Design review of the part shown in the three views and the two pictorial views. Dimensions are in mm from the part's minimum x, y and z. Round coordinates to 2 decimals unless told otherwise and drop trailing zeros. Loops run counter-clockwise (first coordinate to the right, second up) from the corner with the lowest first, then second, coordinate; pieces in that order, holes last. Notation, with made-up numbers: M -4.5,-39 L 42.5,-39 A28 cw 42.5,-17 Z; hole C 84,51.5 d7. An arc over 180 degrees is marked long. One line per question, with ' | ' between items. Start each with the question number.
1) We need section A-A (x = 17.9). Give the boundary of the cut face in (y, z), and give its area (3 significant figures).
2) For pin 1 Ø2 at (x, y) = (13.5, 39.5) entering from -Z; pin 2 Ø2 at (x, y) = (17, 43) entering from -Z; pin 3 Ø5 at (x, z) = (25, 10.5) entering from -Y; pin 4 Ø8 at (x, y) = (31.5, 19.5) entering from +Z, all flat-tipped, find the tip position at first contact; note any pin that passes through.
3) We need section D-D (x = 2). Give the boundary of the cut face in (y, z), and give its area (3 significant figures).
4) For probe 1 along Z at (x, y) = (17.9, 25.5); probe 2 along X at (y, z) = (44, 19); probe 3 along X at (y, z) = (21, 17), list the stretches that pass through material, from the lowest coordinate up. Write a range as from..to.
5) Mouldability with a two-part tool opening along Z and no side actions: class the marked faces 1, 2 and 3 as pulls with the +Z half, pulls with the -Z half, needs draft (parallel to the pull), parting line crosses it, or undercut.
6) We need section C-C (y = 31). Give the boundary of the cut face in (x, z), and give its area (3 significant figures).
7) We need section B-B (z = 17.9). Give the boundary of the cut face in (x, y).
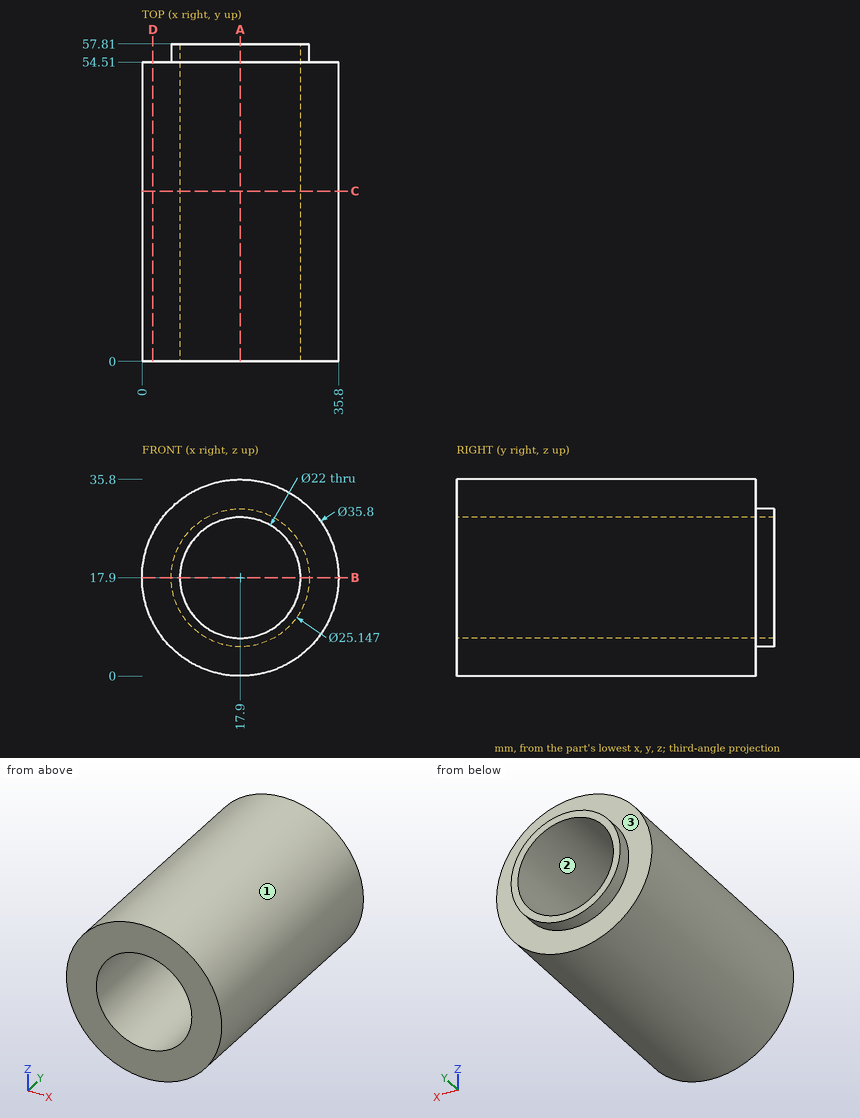
Answers below:
1) outline: M 0,0 L 54.51,0 L 54.51,5.33 L 57.81,5.33 L 57.81,6.9 L 0,6.9 Z; M 0,28.9 L 57.81,28.9 L 57.81,30.47 L 54.51,30.47 L 54.51,35.8 L 0,35.8 Z | area: 763 mm^2
2) pin 1: z = 0.33 | pin 2: z = 0 | pin 3: y = 0 | pin 4: z = 33.01
3) outline: M 0,9.68 L 54.51,9.68 L 54.51,26.12 L 0,26.12 Z | area: 896 mm^2
4) probe 1: 0..6.9, 28.9..35.8 | probe 2: 0.03..6.96, 28.84..35.77 | probe 3: 0.02..6.94, 28.86..35.78
5) face 1: parting line crosses it | face 2: undercut | face 3: needs draft
6) outline: C 17.9,17.9 d35.8; hole C 17.9,17.9 d22 | area: 626 mm^2
7) outline: M 0,0 L 6.9,0 L 6.9,57.81 L 5.33,57.81 L 5.33,54.51 L 0,54.51 Z; M 28.9,0 L 35.8,0 L 35.8,54.51 L 30.47,54.51 L 30.47,57.81 L 28.9,57.81 Z
